CAD build for the part. Positions are in the model's coordinates, mm. A direction names the side the tool comes from. Give positions to 0.01 mm unless a question says otherwise; leave off trailing zeros. Loops run counter-clockwise (first coordinate to the right, second up) from the corner with the lowest first, then second, coordinate; pieces in that order, holes last.
Item 1: Saw through at B-B on z = -116. Give the cut face in (x, y), plus the area to 3 significant figures.
Item 2: Saw through at A-A on y = 15.75. Give the cut face in (x, z).
Item 3: Saw through at C-C on x = 137.5. Give the cut face in (y, z), plus the area to 3 significant figures.
Item 4: Saw through at D-D on z = 137.5. Give the cut face in (x, y), plus the area to 3 significant figures.
Item 5: Probe probe 1 along X at (y, z) = (11.75, 137.5); probe 2 along X at (y, z) = (14, -137.5); probe 3 along Y at (x, z) = (116, -119). List the from-to ranges inside material, lowest first.
Item 6: Drop flat-ended pins along their axis: P1, Ø1.5, axis at y = 11, z = -14, coming from the -X side; P2, Ø9, axis at x = 137.5, z = -137.5, coming from the -Y side; P3, Ø3, axis at x = -139.5, z = 137, coming from the +Y side; P4, Ø1.5, axis at x = 61.5, z = 66.5, coming from the +Y side. Give the stop position or say it passes through.
Item 7: Mould opens along X. For faces 5 (the flat face through (-137, 5, 137)), 6 (the flat face through (-126, 20, -127)), 7 (the flat face through (-150, 8, 2)), 8 (the flat face through (-90, 15, 138)) say: released by +X, released by -X, zero draft, split by the parting line, or undercut.
Item 8: Which spindle directions (+Z, -Z, +X, -X, +Y, -Y) get a long thin tool onto all of the face, cutting with end or side? Do faces 1 (the flat face through (-137, 15, -90)), 2 (the flat face through (-127, 20, 126)), 3 (the flat face through (125, 15, -108)), 4 (the flat face through (90, 15, -138)). Say none if no direction does.
from build123d import *

# Parameters (mm, degrees)
SKETCH1_W           = 300
SKETCH1_H           = 300
BOSS_EXTRUDE1_DEPTH = 10
BOSS_EXTRUDE2_DEPTH = 10
SKETCH3_R           = 5
CUT_EXTRUDE1_DEPTH  = 15


with BuildPart() as part:
    # Sketch1 → Boss-Extrude1 (new body)
    with BuildSketch(Plane(origin=(0, 0, 0), x_dir=(1, 0, 0), z_dir=(0, 1, 0))):
        Rectangle(SKETCH1_W, SKETCH1_H)
    extrude(amount=BOSS_EXTRUDE1_DEPTH)

    # Sketch2 → Boss-Extrude2 (add)
    with BuildSketch(Plane(origin=(0, 10, 0), x_dir=(1, 0, 0), z_dir=(0, 1, 0))):
        Polygon((150, 150), (90, 150), (90, 125), (125, 125), (125, 90), (150, 90), align=None)
        Polygon((-150, 90), (-150, 150), (-90, 150), (-90, 125), (-125, 125), (-125, 90), align=None)
        Polygon((-150, -150), (-90, -150), (-90, -125), (-125, -125), (-125, -90), (-150, -90), align=None)
        Polygon((150, -90), (150, -150), (90, -150), (90, -125), (125, -125), (125, -90), align=None)
    extrude(amount=BOSS_EXTRUDE2_DEPTH)

    # Sketch3 → Cut-Extrude1 (cut)
    with BuildSketch(Plane(origin=(0, 20, 0), x_dir=(1, 0, 0), z_dir=(0, 1, 0))):
        with Locations(Location((-137.5, -137.5, 0), (0, 0, 270))):
            Circle(SKETCH3_R)
        with Locations(Location((137.5, 137.5, 0), (0, 0, 270))):
            Circle(SKETCH3_R)
    extrude(amount=-CUT_EXTRUDE1_DEPTH, mode=Mode.SUBTRACT)


solid = part.part
Results below:
1. outline: (-150, 0) - (150, 0) - (150, 20) - (125, 20) - (125, 10) - (-125, 10) - (-125, 20) - (-150, 20) - close
1. area: 3,500 mm2
2. outline: (-150, -150) - (-90, -150) - (-90, -125) - (-125, -125) - (-125, -90) - (-150, -90) - close; (-150, 90) - (-125, 90) - (-125, 125) - (-90, 125) - (-90, 150) - (-150, 150) - close; (90, -150) - (150, -150) - (150, -90) - (125, -90) - (125, -125) - (90, -125) - close; (90, 125) - (125, 125) - (125, 90) - (150, 90) - (150, 150) - (90, 150) - close; hole circle Ø10 at (-137.5, 137.5); hole circle Ø10 at (137.5, -137.5)
3. outline: (0, -150) - (20, -150) - (20, -142.5) - (5, -142.5) - (5, -132.5) - (20, -132.5) - (20, -90) - (10, -90) - (10, 90) - (20, 90) - (20, 150) - (0, 150) - close
3. area: 4,050 mm2
4. outline: (-150, 0) - (150, 0) - (150, 20) - (90, 20) - (90, 10) - (-90, 10) - (-90, 20) - (-132.5, 20) - (-132.5, 5) - (-142.5, 5) - (-142.5, 20) - (-150, 20) - close
4. area: 4,050 mm2
5. probe 1: x = -150 to -142.5, -132.5 to -90, 90 to 150
5. probe 2: x = -150 to -90, 90 to 132.5, 142.5 to 150
5. probe 3: y = 0 to 10
6. P1: passes through
6. P2: stops at y = 0
6. P3: stops at y = 5
6. P4: stops at y = 10
7. face 5: undercut
7. face 6: zero draft
7. face 7: released by -X
7. face 8: undercut
8. face 1: +X, -X, +Y
8. face 2: +Z, -Z, +X, -X, +Y
8. face 3: +Y
8. face 4: +Z, -Z, +Y
